Source: CAD feature listing. Evaluate the final solid. Frame: model axes, mm. Face numbers are marked on the shaded views. A direction names the side the tool comes from. Round coordinates to 2 decimals unless told otherwise and drop trailing zeros. Order: outer loops, then holes, each group sorted by start corner. A loop starts at its lowest first (then second) coordinate and runs counter-clockwise, first axis right, second up. Notation, with made-up numbers: (82, 58) - (116, 58) arc R10 cw to (116, 74) - close; hole circle Ø6 at (-29, -13). An arc over 180 degrees is marked (long way). Put each result on its own line as item: value. Start each with the question number.
1) Section C-C on x = 0. Output: boundary loops of the cut face in (y, z), then the cut area to 3 significant figures.
2) Line query: probe 1 along X at (y, z) = (33.5, -17); probe 2 along X at (y, z) = (41.5, 5); probe 3 along Y at (x, z) = (0, -20). Output: solid intervals per line, ascending. Write a range as [from, to].
3) Section A-A on x = 33. Output: boundary loops of the cut face in (y, z).
4) Section B-B on y = 50. Output: boundary loops of the cut face in (x, z), then the cut area to 3 significant figures.
5) Mould query, pull axis X, two halves, no side actions, for the marked faces 1, 2, 3 and 4. Classes: +X half, -X half, draft (parallel to the pull), parting line (faces both ways), or undercut.
6) Access query for the marked faces 5, 6, 7, 8 and 9. Directions: +Z, -Z, +X, -X, +Y, -Y. A direction counts if a zero-diameter tool reaches every point of the face in a straight line with its end or side. Return the directions, or none.
7) Contact query for flat-ended pins moving along their axis: P1, Ø6, axis at y = 52, z = 4, coming from the -X side; P2, Ø12, axis at x = 42.5, y = 51, coming from the +Z side; P3, Ø2.5, axis at x = -13.5, z = 3.5, coming from the +Y side; P4, Ø4, axis at y = 39.5, z = -20, coming from the -X side. Output: stop coordinate, or through.
8) Section D-D on y = 24. Output: boundary loops of the cut face in (x, z).
```python
from build123d import *

# Parameters (mm, degrees)
SKETCH1_R            = 5.25
BOSS_EXTRUDE1_DEPTH  = 8
BOSS_EXTRUDE2_DEPTH  = 10
LPATTERN1_COUNT      = 3
LPATTERN1_PITCH      = 56.25
MIRROR1_COPY_1_DEPTH = 10
MIRROR1_COPY_2_DEPTH = 10
CUT_EXTRUDE1_START   = -5
SKETCH3_R            = 15
CUT_EXTRUDE1_DEPTH   = 50


with BuildPart() as part:
    # Sketch1 → Boss-Extrude1 (new body)
    with BuildSketch(Plane.XY):
        with BuildLine():
            Line((51.666666667, 10), (35, 26.666666667))
            Line((35, 26.666666667), (35, 60))
            Line((35, 60), (25, 60))
            Line((25, 60), (25, 26.666666667))
            Line((25, 26.666666667), (16.25, 17.916666667))
            Line((16.25, 17.916666667), (7.5, 26.666666667))
            Line((7.5, 26.666666667), (7.5, 35))
            ThreePointArc((7.5, 35), (0, 42.5), (-7.5, 35))
            Line((-7.5, 35), (-7.5, 26.666666667))
            Line((-7.5, 26.666666667), (-24.166666667, 10))
            Line((-24.166666667, 10), (-37.5, 10))
            Line((-37.5, 10), (-37.5, 0))
            Line((-37.5, 0), (85, 0))
            Line((85, 0), (85, 60))
            Line((85, 60), (75, 60))
            Line((75, 60), (75, 26.666666667))
            Line((75, 26.666666667), (58.333333333, 10))
            Line((58.333333333, 10), (51.666666667, 10))
        make_face()
        Polygon((20.492640687, 13.67402598), (25, 18.181385292), (25, 10), (24.166666667, 10), align=None, mode=Mode.SUBTRACT)
        Polygon((43.181385292, 10), (35, 10), (35, 18.181385292), align=None, mode=Mode.SUBTRACT)
        Polygon((-7.5, 10), (-15.681385292, 10), (-7.5, 18.181385292), align=None, mode=Mode.SUBTRACT)
        Polygon((7.5, 18.181385292), (12.007359313, 13.67402598), (8.333333333, 10), (7.5, 10), align=None, mode=Mode.SUBTRACT)
        Polygon((75, 10), (66.818614708, 10), (75, 18.181385292), align=None, mode=Mode.SUBTRACT)
        with Locations((0, 35)):
            Circle(SKETCH1_R, mode=Mode.SUBTRACT)
    boss_extrude1 = extrude(amount=BOSS_EXTRUDE1_DEPTH)

    # Sketch2 → Boss-Extrude2 (add)
    with BuildSketch(Plane(origin=(-37.5, 0, 0), x_dir=(0, 0, -1), z_dir=(1, 0, 0))):
        Polygon((7.5, 4.166666667), (0, 8.333333333), (0, 0), (7.5, 0), align=None)
    boss_extrude2 = extrude(amount=BOSS_EXTRUDE2_DEPTH)

    # LPattern1: Boss-Extrude2 ×3
    with Locations(*[(i * LPATTERN1_PITCH, 0, 0) for i in range(1, LPATTERN1_COUNT)]):
        add(boss_extrude2)

    # Mirror1: Boss-Extrude1, Boss-Extrude2 across plane
    add(boss_extrude1.mirror(Plane(origin=(-27.5, 0, -7.5), x_dir=(1, 0, 0), z_dir=(0, 0, 1))))
    add(boss_extrude2.mirror(Plane(origin=(-27.5, 0, -7.5), x_dir=(1, 0, 0), z_dir=(0, 0, 1))))

    # Mirror1 copy 1 sketch → Mirror1 copy 1 (add)
    with BuildSketch(Plane(origin=(18.75, 0, -15), x_dir=(0, 0, 1), z_dir=(1, 0, 0))):
        Polygon((7.5, -4.166666667), (0, -8.333333333), (0, 0), (7.5, 0), align=None)
    extrude(amount=MIRROR1_COPY_1_DEPTH)

    # Mirror1 copy 2 sketch → Mirror1 copy 2 (add)
    with BuildSketch(Plane(origin=(75, 0, -15), x_dir=(0, 0, 1), z_dir=(1, 0, 0))):
        Polygon((7.5, -4.166666667), (0, -8.333333333), (0, 0), (7.5, 0), align=None)
    extrude(amount=MIRROR1_COPY_2_DEPTH)

    # Sketch3 → Cut-Extrude1 (cut)
    with BuildSketch(Plane(origin=(35, 0, 0), x_dir=(0, 0, -1), z_dir=(1, 0, 0)).offset(CUT_EXTRUDE1_START)):
        with Locations((7.5, 60)):
            Circle(SKETCH3_R)
    extrude(amount=CUT_EXTRUDE1_DEPTH, mode=Mode.SUBTRACT)


solid = part.part
```
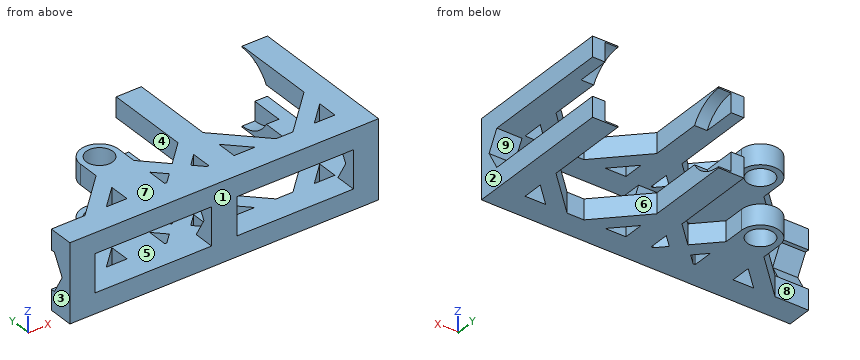
Answer sheet:
1. outline: (0, -23) - (29.75, -23) - (29.75, -15) - (0, -15) - close; (0, 0) - (29.75, 0) - (29.75, 8) - (0, 8) - close; (40.25, -23) - (42.5, -23) - (42.5, -15) - (40.25, -15) - close; (40.25, 0) - (42.5, 0) - (42.5, 8) - (40.25, 8) - close
1. area: 512 mm^2
2. probe 1: [-7.5, -5.03], [5.03, 7.5], [25, 35], [75, 85]
2. probe 2: [-3.74, 3.74], [25, 35], [75, 85]
2. probe 3: [0, 29.75], [40.25, 42.5]
3. outline: (0, -23) - (60, -23) - (60, -22.5) arc R15 cw to (47.01, -15) - (0, -15) - close; (0, 0) - (47.01, 0) arc R15 cw to (60, 7.5) - (60, 8) - (0, 8) - close
4. outline: (25, -23) - (35, -23) - (35, -18.68) - (30, -18.68) - (30, -15) - (25, -15) - close; (25, 0) - (30, 0) - (30, 3.68) - (35, 3.68) - (35, 8) - (25, 8) - close; (75, -23) - (85, -23) - (85, -15) - (80, -15) - (80, -18.68) - (75, -18.68) - close; (75, 3.68) - (80, 3.68) - (80, 0) - (85, 0) - (85, 8) - (75, 8) - close
4. area: 246 mm^2
5. face 1: draft
5. face 2: +X half
5. face 3: -X half
5. face 4: undercut
6. face 5: +Y
6. face 6: +Z, -Z, +Y
6. face 7: +Z, +X, -X, +Y, -Y
6. face 8: +Z, -Z, -X, +Y
6. face 9: +X, -X, +Y
7. P1: x = 25
7. P2: through
7. P3: y = 21.92
7. P4: x = -7.07
8. outline: (-10.17, -23) - (10.17, -23) - (10.17, -15) - (-10.17, -15) - close; (-10.17, 0) - (10.17, 0) - (10.17, 8) - (-10.17, 8) - close; (22.33, -23) - (37.67, -23) - (37.67, -15) - (22.33, -15) - close; (22.33, 0) - (37.67, 0) - (37.67, 8) - (22.33, 8) - close; (72.33, -23) - (85, -23) - (85, -15) - (72.33, -15) - close; (72.33, 0) - (85, 0) - (85, 8) - (72.33, 8) - close
